Verification items for this drawing (mm, ordinates from the low corner). A direction names the side the tool comes from. Round coordinates to 2 decimals unless told otherwise and drop trailing zeros. Loops run counter-clockwise (first coordinate to the right, second up) from the corner with the lowest first, then second, coordinate; pieces in that order, holes last. Notation, with made-up numbers: (88.5, -27.75) -> (95.5, -27.75) arc R26 ccw to (95.5, -10.75) -> close; hole circle Ø2 at (-39, 21). An arc over 180 degrees is marked (long way). One line per item, written item: value. Start each with the question number.
1. Set-up check for the marked faces 1 and 2: record each of +Z, -Z, +X, -X, +Y, -Y from which the full face is reachable in a straight line by a thin tool's end or side.
2. Cross-section at B-B on y = 6.25. Record the cut outline in (x, z).
3. Go/stop test with flat-tipped pins: pin 1 (2 mm diameter, centred on x = 1, y = 8.5, fed in from +Z) (1 decimal); pin 2 (3 mm diameter, centred on y = 9, z = 3.5, fed in from -X); pin 3 (3 mm diameter, centred on x = 3, y = 4.5, fed in from +Z). Record where each tip stops, or that it passes through.
4. Material ranges on L1, parallel to Z at x = 2.9, y = 3.5; L2, parallel to Z at x = 3.4, y = 6.5; L3, parallel to Y at x = 4.2, z = 2.8, recorded low to high.
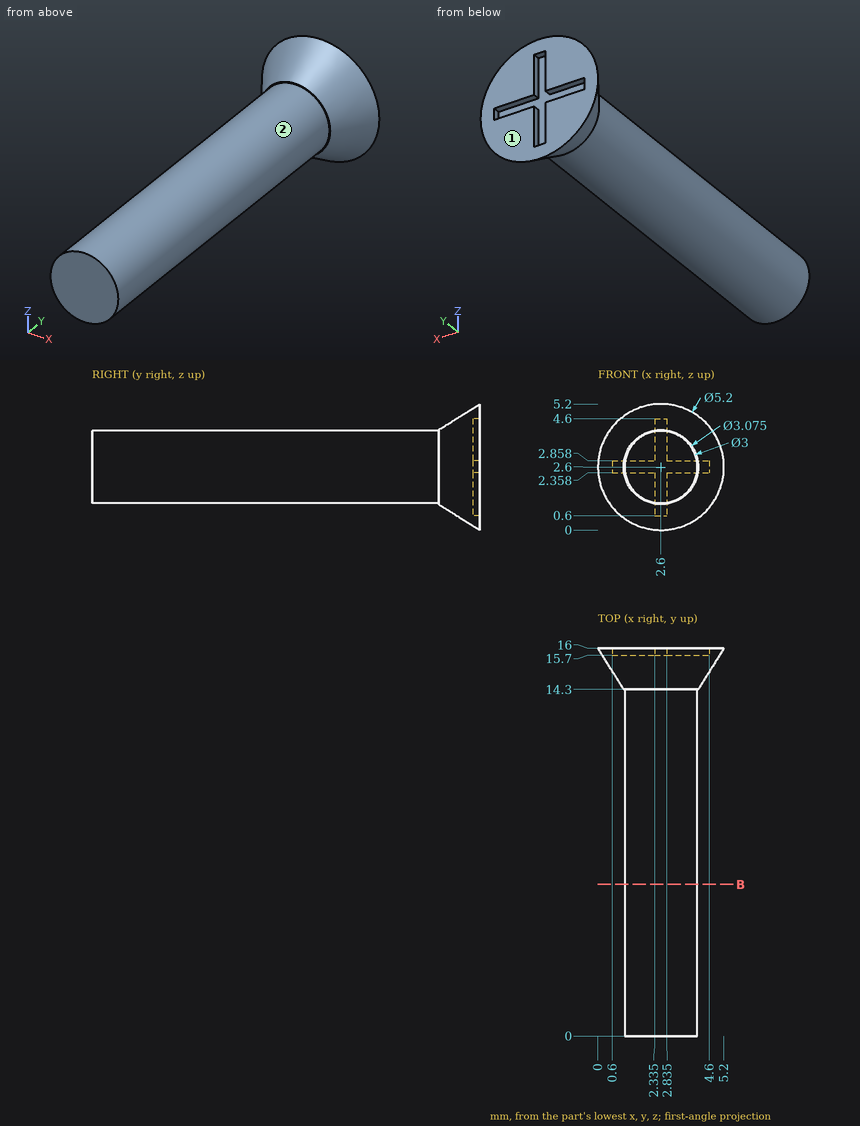
Taken from the geometry:
1. face 1: +Z, -Z, +X, -X, +Y
1. face 2: -Y
2. outline: circle Ø3 at (2.6, 2.6)
3. pin 1: stops at z = 4
3. pin 2: stops at x = 1.1
3. pin 3: stops at z = 4.1
4. L1: z = 1.13 to 4.07
4. L2: z = 1.33 to 3.87
4. L3: y = 14.42 to 15.7
